Geometry check sheet. Reference: drawing and pictorial views, mm from the part's lowest x, y, z. A direction names the side the tool comes from. Round coordinates to 2 decimals unless told otherwise and drop trailing zeros. Loops run counter-clockwise (first coordinate to the right, second up) from the corner with the lowest first, then second, coordinate; pieces in that order, holes last. Notation, with made-up numbers: (28, 10) -> (56, 10) arc R20 cw to (56, 47) -> close; hole circle Ø1 at (36.5, 46). An arc over 180 degrees is marked (long way). Use one line per item in the form item = value. Start each with the question number.
(1) Material ranges on probe 1 along Y at (x, z) = (11, 12.5); probe 2 along Y at (x, z) = (10.75, 5); probe 3 along Z at (x, y) = (16.5, 11), recorded low to high. Write a range as [from, to].
(2) Sectioned sample at D-D (x = 14.25). Record the cut outline in (y, z), and give its area (3 significant figures).
(3) Sectioned sample at C-C (y = 3.25). Record the cut outline in (x, z), and give its area (3 significant figures).
(4) Draft check along X on the marked faces 1, 2 and 3. Enter one of: released by +X, released by -X, zero draft, split by the parting line, or undercut.
(5) Go/stop test with flat-tipped pins: pin 1 (4.5 mm diameter, centred on x = 3.25, y = 11, fed in from -Z); pin 2 (6 mm diameter, centred on x = 10, y = 19, fed in from +Z); pin 3 (1.5 mm diameter, centred on x = 16, z = 4, fed in from -Y). Record where each tip stops, or that it passes through.
(6) Set-up check for the marked faces 4, 5 and 6: record each of +Z, -Z, +X, -X, +Y, -Y from which the full face is reachable in a straight line by a thin tool's end or side.
(7) Sectioned sample at A-A (x = 11). Record the cut outline in (y, z), and give its area (3 significant figures).
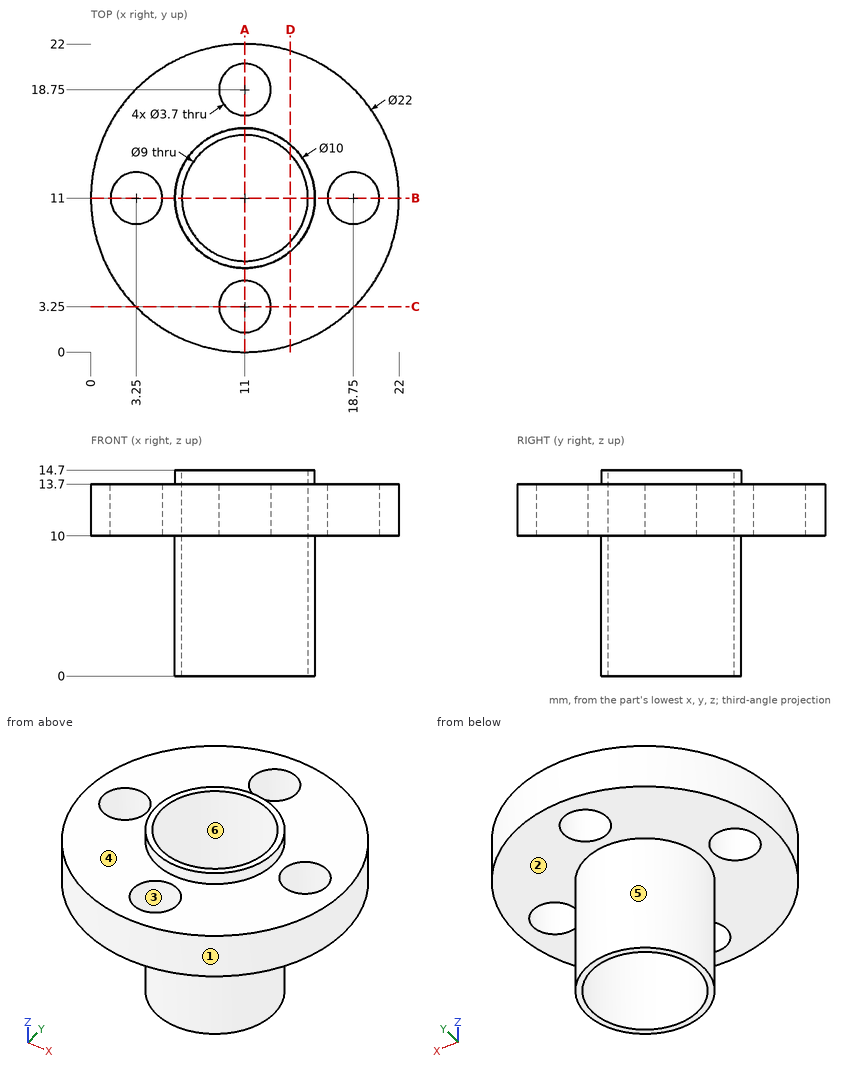
Checks:
q1.probe_1 = [0, 1.4], [5.1, 6.5], [15.5, 16.9], [20.6, 22]
q1.probe_2 = [6.01, 6.51], [15.49, 15.99]
q1.probe_3 = [10, 13.7]
q2.outline = (0.49, 10) -> (7.2, 10) -> (7.2, 0) -> (7.89, 0) -> (7.89, 14.7) -> (7.2, 14.7) -> (7.2, 13.7) -> (0.49, 13.7) -> close; (14.11, 0) -> (14.8, 0) -> (14.8, 10) -> (21.51, 10) -> (21.51, 13.7) -> (14.8, 13.7) -> (14.8, 14.7) -> (14.11, 14.7) -> close
q2.area = 69.9 mm2
q3.outline = (3.19, 10) -> (9.15, 10) -> (9.15, 13.7) -> (3.19, 13.7) -> close; (12.85, 10) -> (18.81, 10) -> (18.81, 13.7) -> (12.85, 13.7) -> close
q3.area = 44.1 mm2
q4.face_1 = split by the parting line
q4.face_2 = zero draft
q4.face_3 = undercut
q5.pin_1 = 10
q5.pin_2 = 13.7
q5.pin_3 = 8.37
q6.face_4 = +Z
q6.face_5 = -Z
q6.face_6 = +Z, -Z
q7.outline = (0, 10) -> (1.4, 10) -> (1.4, 13.7) -> (0, 13.7) -> close; (5.1, 10) -> (6, 10) -> (6, 0) -> (6.5, 0) -> (6.5, 14.7) -> (6, 14.7) -> (6, 13.7) -> (5.1, 13.7) -> close; (15.5, 0) -> (16, 0) -> (16, 10) -> (16.9, 10) -> (16.9, 13.7) -> (16, 13.7) -> (16, 14.7) -> (15.5, 14.7) -> close; (20.6, 10) -> (22, 10) -> (22, 13.7) -> (20.6, 13.7) -> close
q7.area = 31.7 mm2
